```python
from build123d import *

# Parameters (mm, degrees)
F1_DEPTH = 9.5
F2_SIZE2 = 350
F2_SIZE  = 100
F3_R     = 50
F4_SIZE  = 20


with BuildPart() as f1:
    # F0 (on Front) → F1 (new body, symmetric)
    with BuildSketch(Plane.XZ):
        Polygon((0, 250), (-150, 250), (-150, -250), (-120, -250), (-120, -150), (-100, -150), (-100, -250), (0, -250), (100, -250), (100, -150), (120, -150), (120, -250), (150, -250), (150, 250), align=None)
        with BuildLine():
            ThreePointArc((-20, 150), (0, 170), (20, 150))
            Line((20, 150), (20, -100))
            ThreePointArc((20, -100), (0, -120), (-20, -100))
            Line((-20, -100), (-20, 150))
        make_face(mode=Mode.SUBTRACT)
    extrude(amount=F1_DEPTH, both=True)

    # F2
    f2_edges = [f1.edges().sort_by_distance(p)[0] for p in [
        (150, 0, 250),
        (-150, 0, 250),
    ]]
    f2_side = f1.faces().sort_by_distance((0, 0, 250))[0]
    chamfer(f2_edges, length=F2_SIZE, length2=F2_SIZE2, reference=f2_side)

    # F3
    f3_edges = [f1.edges().sort_by_distance(p)[0] for p in [
        (-50, 0, 250),
        (50, 0, 250),
    ]]
    fillet(f3_edges, radius=F3_R)

    # F4
    f4_edges = [f1.edges().sort_by_distance(p)[0] for p in [
        (-150, 0, -250),
        (150, 0, -250),
    ]]
    chamfer(f4_edges, length=F4_SIZE)


solid = f1.part
```
Part model, mm, in its own coordinate system. A direction names the side the tool comes from. Round coordinates to 2 decimals unless told otherwise and drop trailing zeros. Order: outer loops, then holes, each group sorted by start corner. A loop starts at its lowest first (then second) coordinate and runs counter-clockwise, first axis right, second up. Notation, with made-up numbers: M 70.25,85 L 77.25,85 A26 cw 77.25,112 Z; hole C 44.25,52.5 d5. An arc over 180 degrees is marked long. Put each result on its own line as item: value. Start each with the question number.
1. Tool access for faces 5 (the face through (0, 0, 250)), 6 (the face through (110, 0, -150)), 7 (the face through (0, 0, 170)): list every direction of +Z, -Z, +X, -X, +Y, -Y with a clear straight run to the whole face (end or side of a thin tool).
2. Two-plate mould, pull along X, no slides. Class faces 1 (the face through (150, 0, -166)), 2 (the face through (0, 0, -120)), 3 (the face through (-150, 0, -164)), 4 (the face through (120, 0, -199)): +X half, -X half, draft (parallel to the pull), parting line (faces both ways), or undercut.
3. Slice it at C-C on z = 162.5. List the corners of the cut face in (x, y), then the cut area to 3 significant figures.
4. Slice it at A-A on x = 0. List the corners of the cut face in (y, z), then the cut area to 3 significant figures.
5. Slice it at B-B on y = 0.75. List the corners of the cut face in (x, z), then the cut area to 3 significant figures.
6. Drop flat-ended pins along their axis: pin 1 (3 mm diameter, centred on x = 45, y = -2, fed in from +Z); pin 2 (9.5 mm diameter, centred on y = 0.5, z = -20, fed in from +X); pin 3 (2 mm diameter, centred on y = -6.5, z = 174.5, fed in from +X). Give the stop position or say it passes through.
7. Slice it at D-D on x = -87. List the corners of the cut face in (y, z).
8. Drill centre lines: probe 1 along X at (y, z) = (2.5, -187.5); probe 2 along X at (y, z) = (5.75, 63.5); probe 3 along X at (y, z) = (-6, 143). Where is each one in solid material? Low to high. Write a range as [from, to].
Findings:
1. face 5: +Z, +X, -X, +Y, -Y
1. face 6: -Z, +Y, -Y
1. face 7: +Y, -Y
2. face 1: +X half
2. face 2: undercut
2. face 3: -X half
2. face 4: undercut
3. outline: M -75,-9.5 L -15.61,-9.5 L -15.61,9.5 L -75,9.5 Z; M 15.61,-9.5 L 75,-9.5 L 75,9.5 L 15.61,9.5 Z
3. area: 2,260 mm2
4. outline: M -9.5,-250 L 9.5,-250 L 9.5,-120 L -9.5,-120 Z; M -9.5,170 L 9.5,170 L 9.5,250 L -9.5,250 Z
4. area: 3,990 mm2
5. outline: M -150,-230 L -130,-250 L -120,-250 L -120,-150 L -100,-150 L -100,-250 L 100,-250 L 100,-150 L 120,-150 L 120,-250 L 130,-250 L 150,-230 L 150,-100 L 60.36,213.74 A50 ccw 12.28,250 L -12.28,250 A50 ccw -60.36,213.74 L -150,-100 Z; hole M -20,-100 A20 ccw 20,-100 L 20,150 A20 ccw -20,150 Z
5. area: 98,800 mm2
6. pin 1: z = 239.06
6. pin 2: x = 128.5
6. pin 3: x = 71.86
7. outline: M -9.5,-250 L 9.5,-250 L 9.5,120.5 L -9.5,120.5 Z
8. probe 1: [-150, -120], [-100, 100], [120, 150]
8. probe 2: [-103.29, -20], [20, 103.29]
8. probe 3: [-80.57, -20], [20, 80.57]
